Drawing for the job (mm, zero at the part's lowest x, y, z). Coordinates: 2 decimals unless noted, no trailing zeros. Write each loop counter-clockwise with the first axis right and the second up, starting at its lowest first coordinate (ties: lowest second). Pieces come first, ordered by that corner, then holes. Notation, with made-up numbers: (52.25, -25.75) -> (72.25, -25.75) arc R21 cw to (72.25, 13.25) -> close; hole circle Ø3 at (68, 87.25). An arc over 180 degrees is marked (long way). Answer as CSV lines item,"result".
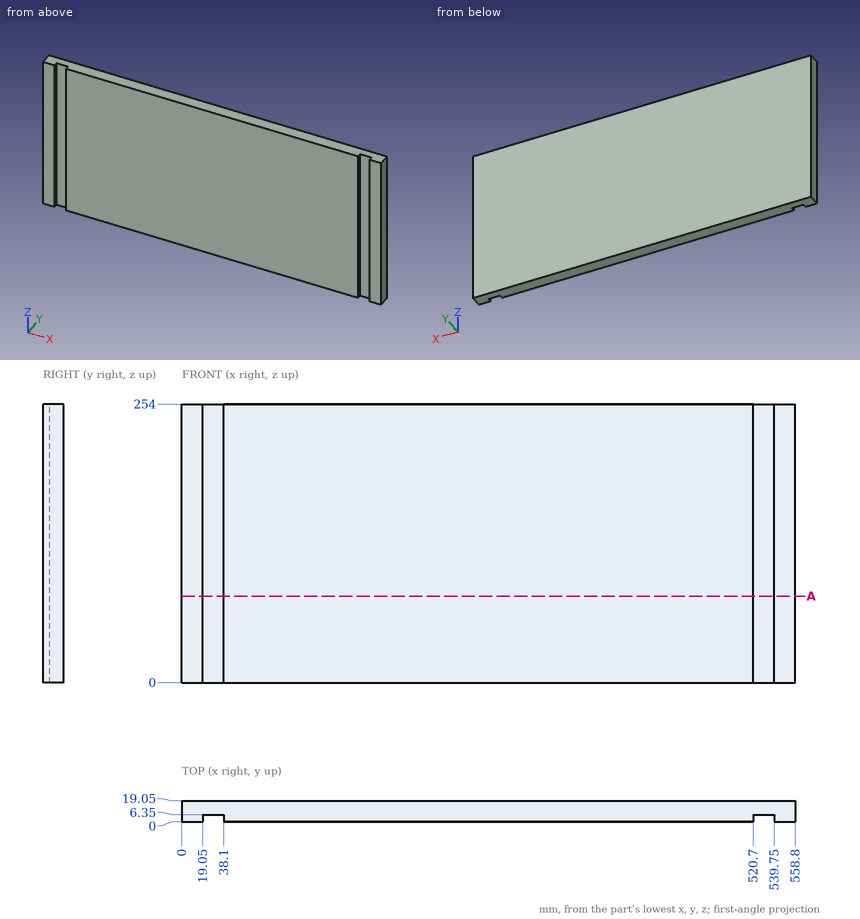
Item 1: Flat gauge pin, fed straight in: pin 1 (5.5 mm diameter, centred on x = 531, z = 153.5, fed in from -Y). Where does the tip first touch, or does it go through?
Answer below:
pin 1,"stops at y = 6.35"
Item 2: Saw through at A-A on z = 79. Give the cut face in (x, y), and give its area (3 significant figures).
Answer below:
outline,"(0, 0) -> (19.05, 0) -> (19.05, 6.35) -> (38.1, 6.35) -> (38.1, 0) -> (520.7, 0) -> (520.7, 6.35) -> (539.75, 6.35) -> (539.75, 0) -> (558.8, 0) -> (558.8, 19.05) -> (0, 19.05) -> close"
area,"10,400 mm2"
Item 3: Wall check: line 1 (X direction, y = 6, z = 23.5). Give the ranges that are in metal, low to high. Write a range as from..to.
Answer below:
line 1,"x = 0..19.05, 38.1..520.7, 539.75..558.8"
